Geometry check sheet. Reference: drawing and pictorial views, mm from the part's lowest x, y, z. A direction names the side the tool comes from. Round coordinates to 2 decimals unless told otherwise and drop trailing zeros. Order: outer loops, then holes, each group sorted by start corner. A loop starts at its lowest first (then second) coordinate and runs counter-clockwise, first axis right, second up.
(1) Release check for a two-part mould opening along Y. For the marked faces 4, 5 and 6 record: +Y half, -Y half, draft (parallel to the pull), parting line (faces both ways), or undercut.
(2) Sectioned sample at D-D (y = 11.75). Record the boundary of the cut face in (x, z).
(3) Set-up check for the marked faces 1, 2 and 3: record each of +Z, -Z, +X, -X, +Y, -Y from which the full face is reachable in a straight line by a thin tool's end or side.
(4) Sectioned sample at A-A (y = 6.5). Record the boundary of the cut face in (x, z).
(5) Sectioned sample at C-C (z = 43.5). Record the boundary of the cut face in (x, y), plus the area to 3 significant figures.
(6) Material ranges on line 1 along Y through (x, z) = (10.6, 1.35); line 2 along Z through (x, y) = (20, 9.75); line 3 along X through (y, z) = (8, 43.5), recorded low to high.
(7) Sectioned sample at B-B (x = 20). Record the boundary of the cut face in (y, z).
(8) Go/stop test with flat-tipped pins: pin 1 (5 mm diameter, centred on x = 26.5, y = 2.5, fed in from -Z); pin 2 (5.5 mm diameter, centred on x = 29.4, y = 6.5, fed in from -Z); pin 3 (4 mm diameter, centred on x = 10.6, y = 6.5, fed in from +Z); pin 4 (3 mm diameter, centred on x = 34.5, y = 3.5, fed in from +Z). Record where each tip stops, or that it passes through.
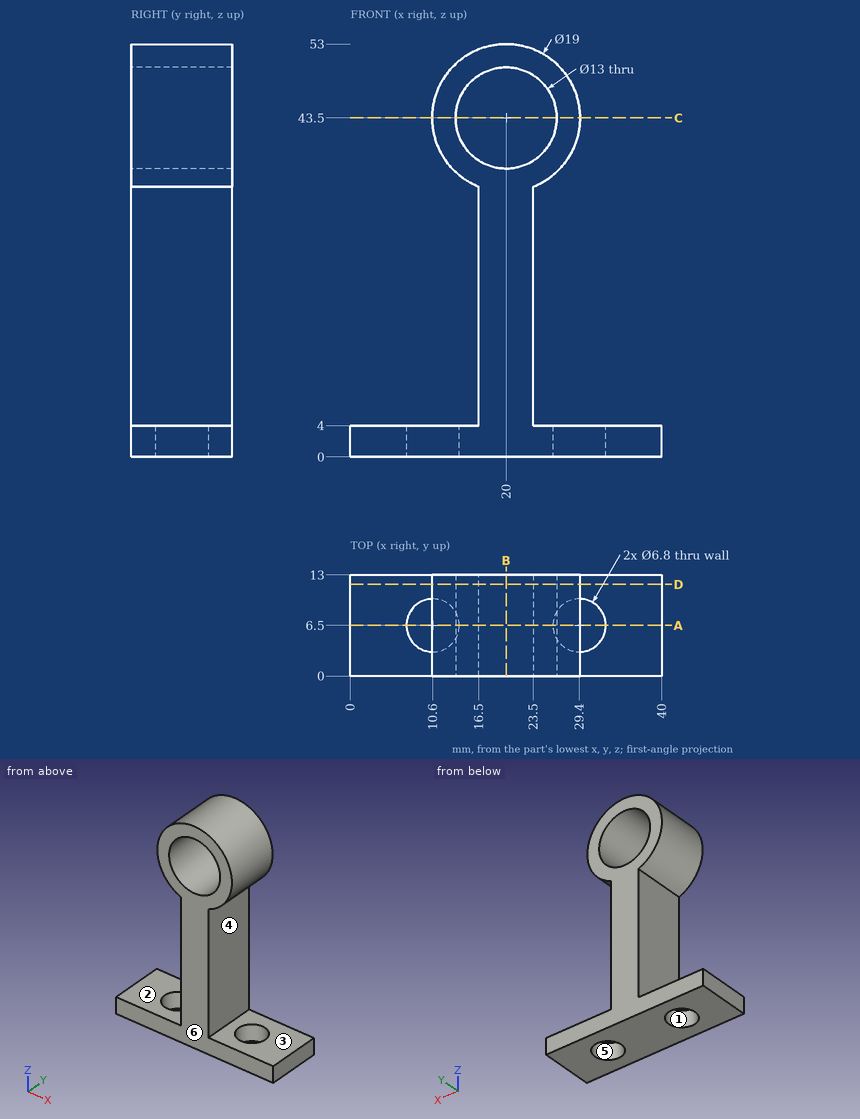
Answer below:
1. face 4: draft
1. face 5: undercut
1. face 6: -Y half
2. outline: (0, 0) - (40, 0) - (40, 4) - (23.5, 4) - (23.5, 34.67) arc R9.5 ccw (long way) to (16.5, 34.67) - (16.5, 4) - (0, 4) - close; hole circle Ø13 at (20, 43.5)
3. face 1: -Z
3. face 2: -X, +Y, -Y
3. face 3: +X, +Y, -Y
4. outline: (0, 0) - (7.2, 0) - (7.2, 4) - (0, 4) - close; (14, 0) - (26, 0) - (26, 4) - (23.5, 4) - (23.5, 34.67) arc R9.5 ccw (long way) to (16.5, 34.67) - (16.5, 4) - (14, 4) - close; (32.8, 0) - (40, 0) - (40, 4) - (32.8, 4) - close; hole circle Ø13 at (20, 43.5)
5. outline: (10.5, 0) - (13.5, 0) - (13.5, 13) - (10.5, 13) - close; (26.5, 0) - (29.5, 0) - (29.5, 13) - (26.5, 13) - close
5. area: 78.0 mm2
6. line 1: y = 0 to 3.1, 9.9 to 13
6. line 2: z = 0 to 37, 50 to 53
6. line 3: x = 10.5 to 13.5, 26.5 to 29.5
7. outline: (0, 0) - (13, 0) - (13, 37) - (0, 37) - close; (0, 50) - (13, 50) - (13, 53) - (0, 53) - close
8. pin 1: stops at z = 0
8. pin 2: stops at z = 36.72
8. pin 3: stops at z = 49.46
8. pin 4: stops at z = 4
